Verification items for this drawing (mm, ordinates from the low corner). Give positions to 0.01 mm unless a question says otherwise; leave off trailing zeros. Loops run counter-clockwise (first coordinate to the right, second up) from the corner with the lowest first, then second, coordinate; pieces in that order, holes last. Notation, with made-up numbers: M 42,72.5 L 68,72.5 A22 cw 68,92.5 Z; hole C 43.5,19 d6. An arc over 180 degrees is marked long. Answer in a Markdown table with one row per item.
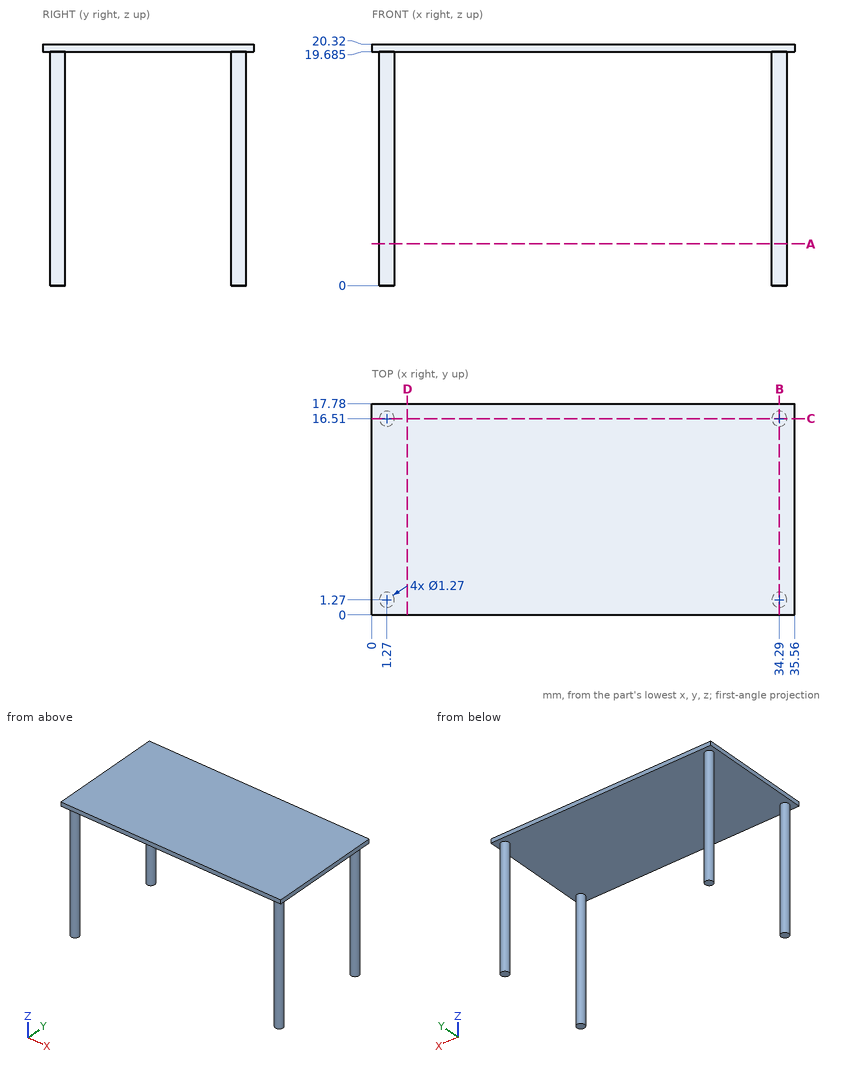
Item 1: Sectioned sample at D-D (x = 3). Record the cut outline in (y, z) (3 decimals).
Reported:
| item | result |
|---|---|
| outline | M 0,19.685 L 17.78,19.685 L 17.78,20.32 L 0,20.32 Z |
Item 2: Sectioned sample at C-C (y = 16.51). Record the cut outline in (x, z) (3 decimals), and give its area (3 significant figures).
Reported:
| item | result |
|---|---|
| outline | M 0,19.685 L 0.635,19.685 L 0.635,0 L 1.905,0 L 1.905,19.685 L 33.655,19.685 L 33.655,0 L 34.925,0 L 34.925,19.685 L 35.56,19.685 L 35.56,20.32 L 0,20.32 Z |
| area | 72.6 mm^2 |
Item 3: Go/stop test with flat-tipped pins: pin 1 (10 mm diameter, centred on y = 15, z = 13, fed in from -X) (3 decimals); pin 2 (10 mm diameter, centred on y = 16, z = 6.5, fed in from +X) (3 decimals); pin 3 (10 mm diameter, centred on x = 6.5, z = 11.5, fed in from -Y); pin 4 (1 mm diameter, centred on x = 11.5, z = 17.5, fed in from +Y). Record where each tip stops, or that it passes through.
Reported:
| item | result |
|---|---|
| pin 1 | stops at x = 0.635 |
| pin 2 | stops at x = 34.925 |
| pin 3 | stops at y = 0.68 |
| pin 4 | passes through |
Item 4: Scan lines: L1, parallel to Z at x = 14, y = 7.25 (3 decimals); L2, parallel to X at y = 16.75, z = 4.25; L3, parallel to X at y = 16, z = 11.75. Record each from-to range of solid material in increasing order. Write a range as [from, to].
Reported:
| item | result |
|---|---|
| L1 | z = [19.685, 20.32] |
| L2 | x = [0.68, 1.86], [33.7, 34.88] |
| L3 | x = [0.89, 1.65], [33.91, 34.67] |
Item 5: Sectioned sample at B-B (x = 34.29). Record the cut outline in (y, z) (3 decimals).
Reported:
| item | result |
|---|---|
| outline | M 0,19.685 L 0.635,19.685 L 0.635,0 L 1.905,0 L 1.905,19.685 L 15.875,19.685 L 15.875,0 L 17.145,0 L 17.145,19.685 L 17.78,19.685 L 17.78,20.32 L 0,20.32 Z |
Item 6: Sectioned sample at A-A (z = 3.5). Record the cut outline in (x, y) (3 decimals).
Reported:
| item | result |
|---|---|
| outline | C 1.27,1.27 d1.27; C 1.27,16.51 d1.27; C 34.29,1.27 d1.27; C 34.29,16.51 d1.27 |
